Could you check a few things on this model? Use its own coordinates, in mm. A direction names the side the tool comes from. Coordinates: 2 decimals unless noted, no trailing zeros. Order: outer loops, then holes, each group sorted by start corner. A loop starts at its lowest first (then second) coordinate and runs counter-clockwise, first axis right, second up. Notation, with made-up numbers: (37.5, 6) -> (59.5, 6) arc R30 cw to (59.5, 31) -> close; hole circle Ø8 at (-15, 83.5). An arc over 180 degrees is marked (long way). Use a Markdown table: item, result. Add a question column.
1) Which directions (+Z, -Z, +X, -X, +Y, -Y) give clear straight access to the entire face, cutting with the end or side of a thin tool? Please do faces 4 (the flat face through (0, -1, 0)), 5 (the flat face through (-3.5, -1, -0.75)), 6 (the flat face through (3, -2, 1)), 7 (the flat face through (3.5, -1, -0.75)).
2) If we section it at B-B (x = 2.25): Write out the boundary of the cut face in (y, z).
3) If I drill on L1, parallel to X at y = -3.15, z = 0; L2, parallel to Y at x = -1, z = 2; L3, parallel to Z at x = 0, y = -3, over which ranges is the centre line in solid material (lowest first)? Write a range as [from, to].
4) If we section it at C-C (y = -0.5): Write out the boundary of the cut face in (x, z), plus the area to 3 significant figures.
5) If we section it at A-A (z = 0.25): Write out the boundary of the cut face in (x, y), plus the area to 3 significant figures.
6) If we section it at D-D (z = 2): Write out the boundary of the cut face in (x, y), plus the area to 3 significant figures.
7) Will these pins go through, and if not, where does the flat tip stop? pin 1 Ø3.5 at (x, z) = (0, 0) entering from -Y; pin 2 Ø3 at (x, y) = (-2, -2.5) entering from -Z; pin 3 Ø1.6 at (x, z) = (-3, 0.5) entering from +Y; pin 4 Ø1 at (x, y) = (-1, -2) entering from +Z.
8) Thinking about a two-plate mould opening in Z: for faces 1 (the cylindrical face through (0.08, -0.49, 3.95)), 2 (the flat face through (-1, -6.5, -3)), 3 (the cylindrical face through (0, -4, -3)), which applies, +Z half, -Z half, draft (parallel to the pull), parting line (faces both ways), or undercut?
```python
from build123d import *

# Parameters (mm, degrees)
F4_R      = 3.95
F4_R_2    = 3
F5_DEPTH  = 6.5
F6_DEPTH  = 1
F7_W      = 4
F7_H      = 5.5
F8_DEPTH  = 3.951
F10_DEPTH = 1.5
F12_W     = 1
F12_H     = 4.7
F13_DEPTH = 7.901


with BuildPart() as f5:
    # F4 (on Front) → F5 (new body)
    with BuildSketch(Plane.XZ):
        Circle(F4_R)
        Circle(F4_R_2, mode=Mode.SUBTRACT)
    extrude(amount=F5_DEPTH)

    # F4 (on Front) → F6 (join)
    with BuildSketch(Plane.XZ):
        Circle(F4_R_2)
    extrude(amount=F6_DEPTH)

    # F7 (on Top) → F8 (cut, through all)
    with BuildSketch(Plane.XY):
        with Locations((0, -3.75)):
            Rectangle(F7_W, F7_H)
    extrude(amount=F8_DEPTH, mode=Mode.SUBTRACT)

    # F9 (on face) → F10 (cut)
    with BuildSketch(Plane(origin=(0, 0, 0), x_dir=(-1, 0, 0), z_dir=(0, 1, 0))):
        with BuildLine():
            Line((-3.2, 0.75), (-3.8781438859, 0.75))
            ThreePointArc((-3.8781438859, 0.75), (-3.95, 0), (-3.8781438859, -0.75))
            Line((-3.8781438859, -0.75), (-3.2, -0.75))
            ThreePointArc((-3.2, -0.75), (-2.45, 0), (-3.2, 0.75))
        make_face()
        with BuildLine():
            ThreePointArc((3.95, 0), (3.9319949357, 0.3767171688), (3.8781438859, 0.75))
            Line((3.8781438859, 0.75), (3.2, 0.75))
            ThreePointArc((3.2, 0.75), (2.45, 0), (3.2, -0.75))
            Line((3.2, -0.75), (3.8781438859, -0.75))
            ThreePointArc((3.8781438859, -0.75), (3.9319949357, -0.3767171688), (3.95, 0))
        make_face()
    extrude(amount=-F10_DEPTH, mode=Mode.SUBTRACT)

    # F12 (on offset) → F13 (cut, through all)
    with BuildSketch(Plane.YZ.offset(3.95)):
        with Locations((-1.5, 1.6)):
            Rectangle(F12_W, F12_H)
    extrude(amount=-F13_DEPTH, mode=Mode.SUBTRACT)


solid = f5.part
```
Answer sheet:
| question | item | result |
|---|---|---|
| 1 | face 4 | +Z |
| 1 | face 5 | -X |
| 1 | face 6 | +Z, +X, -X |
| 1 | face 7 | +X |
| 2 | outline | (-6.5, -3.25) -> (0, -3.25) -> (0, 3.25) -> (-1, 3.25) -> (-1, -1.98) -> (-6.5, -1.98) -> close; (-6.5, 1.98) -> (-2, 1.98) -> (-2, 3.25) -> (-6.5, 3.25) -> close |
| 3 | L1 | [-3.95, -3], [3, 3.95] |
| 3 | L2 | [-1, 0] |
| 3 | L3 | [-3.95, -3] |
| 4 | outline | (-3.88, -0.75) arc R3.95 ccw to (3.88, -0.75) -> (3.2, -0.75) arc R0.75 cw to (3.2, 0.75) -> (3.88, 0.75) arc R3.95 ccw to (-3.88, 0.75) -> (-3.2, 0.75) arc R0.75 cw to (-3.2, -0.75) -> close |
| 4 | area | 45.1 mm2 |
| 5 | outline | (-3.94, -6.5) -> (-2.99, -6.5) -> (-2.99, -2) -> (-3.94, -2) -> close; (-2.49, -1) -> (2.49, -1) -> (2.49, 0) -> (-2.49, 0) -> close; (2.99, -6.5) -> (3.94, -6.5) -> (3.94, -2) -> (2.99, -2) -> close |
| 5 | area | 13.6 mm2 |
| 6 | outline | (-3.41, -6.5) -> (-2.24, -6.5) -> (-2.24, -2) -> (-3.41, -2) -> close; (-3.41, -1) -> (3.41, -1) -> (3.41, 0) -> (-3.41, 0) -> close; (2.24, -6.5) -> (3.41, -6.5) -> (3.41, -2) -> (2.24, -2) -> close |
| 6 | area | 17.3 mm2 |
| 7 | pin 1 | y = -1 |
| 7 | pin 2 | z = -3.92 |
| 7 | pin 3 | y = 0 |
| 7 | pin 4 | z = -2.6 |
| 8 | face 1 | +Z half |
| 8 | face 2 | draft |
| 8 | face 3 | undercut |
